from build123d import *

# Parameters (mm, degrees)
SKETCH1_R           = 4
BOSS_EXTRUDE1_DEPTH = 73
SKETCH2_R           = 3.2
BOSS_EXTRUDE2_DEPTH = 73
CHAMFER1_SIZE       = 0.5


with BuildPart() as part:
    # Sketch1 → Boss-Extrude1 (new body)
    with BuildSketch(Plane.XY):
        Circle(SKETCH1_R)
    extrude(amount=BOSS_EXTRUDE1_DEPTH)

    # Sketch2 → Boss-Extrude2 (add)
    with BuildSketch(Plane.XY.offset(73)):
        Circle(SKETCH2_R)
    extrude(amount=BOSS_EXTRUDE2_DEPTH)

    # Chamfer1
    chamfer1_edges = [part.edges().sort_by_distance(p)[0] for p in [
        (-4, 0, 0),
        (-3.2, 0, 146),
    ]]
    chamfer(chamfer1_edges, length=CHAMFER1_SIZE)


solid = part.part
Verification items for the finished model (mm, model axes). A direction names the side the tool comes from. Coordinates: 2 decimals unless noted, no trailing zeros. Order: outer loops, then holes, each group sorted by start corner. A loop starts at its lowest first (then second) coordinate and runs counter-clockwise, first axis right, second up. Notation, with made-up numbers: (48.25, 6.5) -> (107.25, 6.5) arc R24 ccw to (107.25, 27.5) -> close; hole circle Ø4 at (75, 62). An arc over 180 degrees is marked (long way). Use CSV: the item, a comma, the result in double quotes. Start each with the question number.
Q1. Section check D-D, the plane z = 38. Record the cut outline in (x, y), and give its area (3 significant figures).
Q2. Depth check by flat-ended pin: P1, Ø1.5, axis at x = 3, y = -0.5, coming from the -Z side. Enter the tip coordinate at first touch or a pass-through.
Q3. Section check C-C, the plane z = 134. Record the cut outline in (x, y), and give its area (3 significant figures).
Q4. Thickness scan on line 1 along X through (y, z) = (0.25, 78); line 2 along X through (y, z) = (0.25, 17.5); line 3 along Y through (x, z) = (1.5, 24). Record the ranges inside material, lowest first.
Q5. Section check A-A, the plane y = 0. Record the cut outline in (x, z).
Q6. Tool access check on faces 1 (the flat face through (-2, 3, 73)), 2 (the flat face through (0, 0, 146)). Record the directions out of +Z, -Z, +X, -X, +Y, -Y that give a thin tool (end or side, any length) a straight path to the whole face; none if there is none.
Returned:
1,outline,"circle Ø8 at (0, 0)"
1,area,"50.3 mm^2"
2,P1,"stops at z = 0"
3,outline,"circle Ø6.4 at (0, 0)"
3,area,"32.2 mm^2"
4,line 1,"x = -3.19 to 3.19"
4,line 2,"x = -3.99 to 3.99"
4,line 3,"y = -3.71 to 3.71"
5,outline,"(-4, 0.5) -> (-3.5, 0) -> (3.5, 0) -> (4, 0.5) -> (4, 73) -> (3.2, 73) -> (3.2, 145.5) -> (2.7, 146) -> (-2.7, 146) -> (-3.2, 145.5) -> (-3.2, 73) -> (-4, 73) -> close"
6,face 1,"+Z"
6,face 2,"+Z, +X, -X, +Y, -Y"
